Model file for the job. Use its own axes, mm. A direction names the side the tool comes from. Give positions to 0.01 mm unless a question says otherwise; leave off trailing zeros. Write each loop counter-clockwise with the first axis right and the second up, starting at its lowest first coordinate (ties: lowest second). Pieces come first, ordered by that corner, then holes.
```python
from build123d import *

# Parameters (mm, degrees)
F0_R     = 69.85
F0_R_2   = 57.15
F1_DEPTH = 203.2
F2_R     = 57.15
F3_DEPTH = 12.7
F4_DEPTH = 203.2


with BuildPart() as f1:
    # F0 (on Front) → F1 (new body)
    with BuildSketch(Plane.XZ):
        Circle(F0_R)
        Circle(F0_R_2, mode=Mode.SUBTRACT)
    extrude(amount=F1_DEPTH)

    # F2 (on Front) → F3 (join)
    with BuildSketch(Plane.XZ):
        Circle(F2_R)
    extrude(amount=F3_DEPTH)

    # F2 (on Front) → F4 (join)
    with BuildSketch(Plane.XZ):
        Circle(F2_R)
    extrude(amount=-F4_DEPTH)


solid = f1.part
```
1. Slice it at B-B, the plane z = 0. Write the cut outline in (x, y), and give its area (3 significant figures).
Calculated:
outline: (-69.85, -203.2) - (-57.15, -203.2) - (-57.15, -12.7) - (57.15, -12.7) - (57.15, -203.2) - (69.85, -203.2) - (69.85, 0) - (57.15, 0) - (57.15, 203.2) - (-57.15, 203.2) - (-57.15, 0) - (-69.85, 0) - close
area: 29,800 mm2
2. Pin check, flat tips, straight feed: P1, Ø8, axis at x = -45.5, z = 49.5, coming from the +Y side; P2, Ø10, axis at y = 150.5, z = -46.5, coming from the +X side; P3, Ø1, axis at y = -0.5, z = 19, coming from the +X side. Stop position of each tip, or through.
Calculated:
P1: stops at y = 0
P2: stops at x = 39.29
P3: stops at x = 67.36
3. Which spindle directions (+Z, -Z, +X, -X, +Y, -Y) get a long thin tool onto all of the face, cutting with end or side? Do faces 1 (the flat face through (-1, -12.7, 1)), 2 (the flat face through (-1, 203.2, 1)). Say none if no direction does.
Calculated:
face 1: -Y
face 2: +Z, -Z, +X, -X, +Y
4. Slice it at A-A, the plane x = 0. Write the cut outline in (y, z), and give its area (3 significant figures).
Calculated:
outline: (-203.2, -69.85) - (0, -69.85) - (0, -57.15) - (203.2, -57.15) - (203.2, 57.15) - (0, 57.15) - (0, 69.85) - (-203.2, 69.85) - (-203.2, 57.15) - (-12.7, 57.15) - (-12.7, -57.15) - (-203.2, -57.15) - close
area: 29,800 mm2
5. Pull direction Z, two halves, no side cores. Call faces 3 (the cylindrical face through (-57.095, 100.178, 2.513)), 4 (the cylindrical face through (-57.095, -106.616, 2.513)), 5 (the flat face through (-26.2, 0, -51.4)): +Z half, -Z half, draft (parallel to the pull), parting line (faces both ways), or undercut.
Calculated:
face 3: parting line
face 4: undercut
face 5: draft
6. Slice it at D-D, the plane y = -69.5. Write the cut outline in (x, z).
Calculated:
outline: circle Ø139.7 at (0, 0); hole circle Ø114.3 at (0, 0)
7. Slice it at C-C, the plane y = 120. Write the cut outline in (x, z), and give its area (3 significant figures).
Calculated:
outline: circle Ø114.3 at (0, 0)
area: 10,300 mm2
8. Probe probe 1 along Z at (x, y) = (0, -109.5); probe 2 along Y at (x, z) = (26, 30); probe 3 along Z at (x, y) = (-34.5, -181.5). List the from-to ranges inside material, lowest first.
Calculated:
probe 1: z = -69.85 to -57.15, 57.15 to 69.85
probe 2: y = -12.7 to 203.2
probe 3: z = -60.74 to -45.56, 45.56 to 60.74
